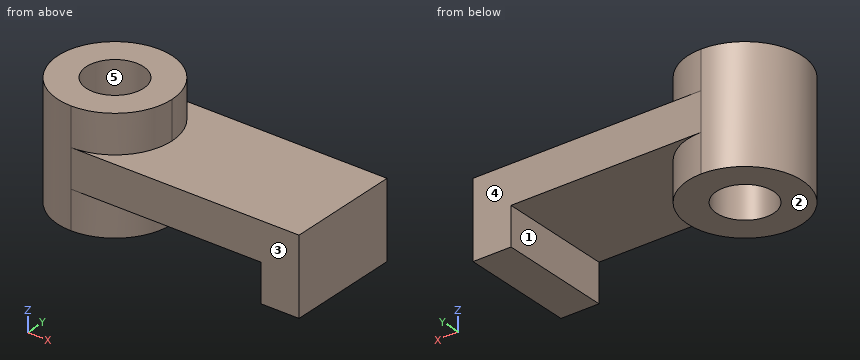
```python
from build123d import *

# Parameters (mm, degrees)
F0_R     = 9.525
F1_DEPTH = 19.05
F2_DEPTH = 6.35
F3_W     = 12.7
F3_H     = 38.1
F4_DEPTH = 12.7


with BuildPart() as f1:
    # F0 (on Top) → F1 (new body, symmetric)
    with BuildSketch(Plane.XY):
        with BuildLine():
            ThreePointArc((-38.1, 19.05), (-57.15, 0), (-38.1, -19.05))
            ThreePointArc((-38.1, -19.05), (-24.629616, -13.470384), (-19.05, 0))
            ThreePointArc((-19.05, 0), (-24.629616, 13.470384), (-38.1, 19.05))
        make_face()
        with Locations((-38.1, 0)):
            Circle(F0_R, mode=Mode.SUBTRACT)
    extrude(amount=F1_DEPTH, both=True)

    # F0 (on Top) → F2 (join, symmetric)
    with BuildSketch(Plane.XY):
        with BuildLine():
            Line((-38.1, -19.05), (38.1, -19.05))
            Line((38.1, -19.05), (38.1, 19.05))
            Line((38.1, 19.05), (-38.1, 19.05))
            ThreePointArc((-38.1, 19.05), (-24.629616, 13.470384), (-19.05, 0))
            ThreePointArc((-19.05, 0), (-24.629616, -13.470384), (-38.1, -19.05))
        make_face()
    extrude(amount=F2_DEPTH, both=True)

    # F3 (on face) → F4 (join)
    with BuildSketch(Plane(origin=(0, 0, -6.35), x_dir=(1, 0, 0), z_dir=(0, 0, -1))):
        with Locations((31.75, 0)):
            Rectangle(F3_W, F3_H)
    extrude(amount=F4_DEPTH)


solid = f1.part
```
Work out the finished part from the listing and answer in its coordinate system (mm). Face numbers are marked on the shaded views. A direction names the side the tool comes from. Round coordinates to 2 decimals unless told otherwise and drop trailing zeros. Order: outer loops, then holes, each group sorted by start corner. A loop starts at its lowest first (then second) coordinate and runs counter-clockwise, first axis right, second up.
Q1. Given pin 1 Ø6.5 at (y, z) = (3.5, -12.5) entering from -X; pin 2 Ø6 at (y, z) = (5, -11) entering from -X; pin 3 Ø19 at (x, y) = (6.5, -9) entering from -Z, each flat-ended and moving along its own axis, determine where each tip first touches the part or whether it passes through.
Solution:
pin 1: stops at x = -57.15
pin 2: stops at x = -57.04
pin 3: stops at z = -6.35
Q2. The mould has two halves that part along Y. Classify the marked faces 3, 4 and 5: pulls with the +Y half, pulls with the -Y half, needs draft (parallel to the pull), parting line crosses it, or undercut.
Solution:
face 3: pulls with the -Y half
face 4: pulls with the +Y half
face 5: undercut
Q3. A cutting plane is placed at D-D, the plane y = 1.5. Determine the outline of the cut face in (x, z).
Solution:
outline: (-57.09, -19.05) - (-47.51, -19.05) - (-47.51, 19.05) - (-57.09, 19.05) - close; (-28.69, -19.05) - (-19.11, -19.05) - (-19.11, -6.35) - (25.4, -6.35) - (25.4, -19.05) - (38.1, -19.05) - (38.1, 6.35) - (-19.11, 6.35) - (-19.11, 19.05) - (-28.69, 19.05) - close
Q4. A cutting plane is placed at B-B, the plane y = 8. Determine the outline of the cut face in (x, z), then the cut area to 3 significant figures.
Solution:
outline: (-55.39, -19.05) - (-43.27, -19.05) - (-43.27, 19.05) - (-55.39, 19.05) - close; (-32.93, -19.05) - (-20.81, -19.05) - (-20.81, -6.35) - (25.4, -6.35) - (25.4, -19.05) - (38.1, -19.05) - (38.1, 6.35) - (-20.81, 6.35) - (-20.81, 19.05) - (-32.93, 19.05) - close
area: 1,830 mm2
Q5. A tool of negligible diameter and unlimited length cuts with its end or side. For the marked faces 1 and 2, from which of +Z, -Z, +X, -X, +Y, -Y can it reach the whole face along a straight path? Write none if from no direction.
Solution:
face 1: -Z, +Y, -Y
face 2: -Z, +X, -X, +Y, -Y
Q6. Find the intervals of material crossed by line 1 along Y through (x, z) = (-38.1, -4) (3 decimals); line 2 along Z through (x, y) = (-2.5, -12), in increasing order.
Solution:
line 1: y = -19.05 to -9.525, 9.525 to 19.05
line 2: z = -6.35 to 6.35
Q7. A cutting plane is placed at C-C, the plane z = 2. Determine the outline of the cut face in (x, y) (3 decimals), then the cut area to 3 significant figures.
Solution:
outline: (-38.1, -19.05) - (38.1, -19.05) - (38.1, 19.05) - (-38.1, 19.05) arc R19.05 ccw to start; hole circle Ø19.05 at (-38.1, 0)
area: 3,190 mm2
Q8. A cutting plane is placed at A-A, the plane z = -10. Determine the outline of the cut face in (x, y) (3 decimals), then the cut area to 3 significant figures.
Solution:
outline: (-38.1, -19.05) arc R19.05 ccw to (-19.05, 0) arc R19.05 ccw (long way) to start; (25.4, -19.05) - (38.1, -19.05) - (38.1, 19.05) - (25.4, 19.05) - close; hole circle Ø19.05 at (-38.1, 0)
area: 1,340 mm2
